Autodesk Fusion 360 part; units mm, degrees
sketch "Sketch1" plane through (0, 0, 0) normal (0, 1, 0) x (1, 0, 0)
  circle A0 centre (0, 0) radius 12.75
  circle A1 centre (0, 0) radius 15.75
  line L0 (0, 0) -> (0, 15.75)
  line L1 (24, 10.75) -> (24, 15.75)
  line L2 (24, 15.75) -> (0, 15.75)
  line L3 (11.5109, 10.75) -> (24, 10.75)
  line L4 (0, 12.75) -> (0, 15.75)
  line L5 (5.5761, 11.466) -> (6.606, 14.2976)
  line L6 (-5.5761, 11.466) -> (-6.606, 14.2976)
  line L7 (6.606, 14.2976) -> (7.1343, 15.75)
  dimension "d1" = 25.5
  dimension "d2" = 3
  dimension "d3" = 24
  dimension "d4" = 5
  dimension "d5" = 12.4891
extrude "Extrude1" add sketch "Sketch1" along normal blind 8 contours A0 A1 L5 L6 makes body 1
extrude "Extrude2" add sketch "Sketch1" along normal blind 8 separate body contours A1 L1 L2 L3 L7 makes body 2
sketch "Sketch2" plane through (0, 0, -10.75) normal (0, 0, 1) x (1, 0, 0)
  line L0 (11.5109, 0) -> (24, 0)
  line L1 (24, 0) -> (24, 8)
  line L2 (24, 8) -> (11.5109, 8)
  line L3 (11.5109, 8) -> (11.5109, 0)
  circle A0 centre (20, 4) radius 3
  circle A1 centre (20, 4) radius 1.9
  line L4 (0, 0) -> (0, 7)
  line L5 (24, 4) -> (20, 4)
  dimension "d10" = 20
  dimension "d11" = 3.8
  dimension "d12" = 6
extrude "Extrude3" cut sketch "Sketch2" against normal blind 9 contours A1 bodies 2
extrude "Extrude4" cut sketch "Sketch2" against normal blind 3 contours A0 bodies 2
mirror "Mirror1" about plane through (0, 0, 0) normal (1, 0, 0) of bodies 2 makes body 3
combine "Combine1" operation add target body 3 tool bodies 1 2
fillet "Fillet1" radius 2.5 6 edges at (11.5109, 4, -10.75) (-11.5109, 4, -10.75) (-5.5761, 4, -11.466) (5.5761, 4, -11.466) (7.1343, 4, -15.75) (-7.1343, 4, -15.75) on bodies 3
chamfer "Chamfer1" distance 0.5 angle 45 28 edges at (0, 8, 15.75) (14.1486, 8, -9.5586) (20.1394, 8, -10.75) (-20.1394, 8, -10.75) (-14.1486, 8, -9.5586) (0, 8, 12.75) (-6.2564, 8, -11.8057) (-6.4118, 8, -13.7636) (-7.451, 8, -15.2977) (-16.4426, 8, -15.75) (16.4426, 8, -15.75) (7.451, 8, -15.2977) (6.4118, 8, -13.7636) (6.2564, 8, -11.8057) (0, 0, 15.75) (14.1486, 0, -9.5586) (20.1394, 0, -10.75) (-20.1394, 0, -10.75) (-14.1486, 0, -9.5586) (0, 0, 12.75) (6.2564, 0, -11.8057) (6.4118, 0, -13.7636) (7.451, 0, -15.2977) (16.4426, 0, -15.75) (-16.4426, 0, -15.75) (-7.451, 0, -15.2977) (-6.4118, 0, -13.7636) (-6.2564, 0, -11.8057) 2 faces at (-24, 5.3333, -12.4167) (-24, 5.3333, -12.4167) on bodies 3
equation "d15 = -5.00 mm + 2 mm"
Design review of the part built by this model. Coordinates are the model's own, in mm. A direction names the side the tool comes from. Round coordinates to 2 decimals unless told otherwise and drop trailing zeros. Loops run counter-clockwise (first coordinate to the right, second up) from the corner with the lowest first, then second, coordinate; pieces in that order, holes last. Notation, with made-up numbers: M -6.5,74.5 L 38.5,74.5 A20 ccw 38.5,89.5 Z; hole C -11,81 d8. An arc over 180 degrees is marked long. Answer as a JSON object with one key per item and string values.
Item 1: Clearance check with flat-ended pins moving along their axes: P1, Ø1.5, axis at y = 3, z = -6.5, coming from the -X side; P2, Ø3, axis at x = -19, y = 4, coming from the +Z side; P3, Ø3, axis at x = 21.5, y = 4.5, coming from the +Z side. State where each tip first meets the part, or that it passes through.
Answer sheet:
{"P1": "stops at x = -14.66", "P2": "stops at z = -13.75", "P3": "stops at z = -10.75"}
Item 2: Machinability: for faces 5 (the cylindrical face through (-6.263, 4.049, -11.784)), 6 (the flat face through (-19.9, 0.8, -10.75)), 7 (the flat face through (23, 6, -10.75)), which of the approach directions +Z, -Z, +X, -X, +Y, -Y give a long, thin tool a straight path to every point of the face, cutting with its end or side? Answer none if there is none.
Answer sheet:
{"face 5": "+Y, -Y", "face 6": "+Z, -X, +Y, -Y", "face 7": "+Z, +X, +Y, -Y"}
Item 3: We need section B-B on x = 0. Give the boundary of the cut face in (y, z), and give its area (3 significant figures).
Answer sheet:
{"outline": "M 0,13.25 L 0.5,12.75 L 7.5,12.75 L 8,13.25 L 8,15.25 L 7.5,15.75 L 0.5,15.75 L 0,15.25 Z", "area": "23.5 mm^2"}
Item 4: We need section C-C on y = 4. State how many separate pieces and enclosed holes the cut face has, and give its area (3 significant figures).
Answer sheet:
{"separate pieces": "3", "enclosed holes": "0", "area": "339 mm^2"}
Item 5: Wall thickness on L1, parallel to X at y = 7, z = 0; L2, parallel to Y at x = 20, z = -14.85; L3, parallel to X at y = 6.5, z = 9: over which ranges is each line inside the solid? List them lowest first. Write a range as from..to.
Answer sheet:
{"L1": "x = -15.75..-12.75, 12.75..15.75", "L2": "y = 0..2.1, 5.9..8", "L3": "x = -12.93..-9.03, 9.03..12.93"}
Item 6: The part is to be moulded in two halves that separate along Y. For faces 1 (the cylindrical face through (0.453, 3.951, 12.742)), 2 (the cylindrical face through (-18.6, 2.716, -14.736)), 3 (the cylindrical face through (17, 4, -12)), 4 (the flat face through (-7, 0, -12)), say which applies: pulls with the +Y half, pulls with the -Y half, needs draft (parallel to the pull), parting line crosses it, or undercut.
Answer sheet:
{"face 1": "needs draft", "face 2": "undercut", "face 3": "undercut", "face 4": "pulls with the -Y half"}
Item 7: We need section A-A on z = 0. Give the boundary of the cut face in (x, y).
Answer sheet:
{"outline": "M -15.75,0.5 L -15.25,0 L -13.25,0 L -12.75,0.5 L -12.75,7.5 L -13.25,8 L -15.25,8 L -15.75,7.5 Z; M 12.75,0.5 L 13.25,0 L 15.25,0 L 15.75,0.5 L 15.75,7.5 L 15.25,8 L 13.25,8 L 12.75,7.5 Z"}
